For this review, take the finished solid that the model builds, in its own axes (mm). A direction names the side the tool comes from. Coordinates: 2 decimals unless noted, no trailing zeros. Write each loop counter-clockwise with the first axis right and the second up, starting at its lowest first coordinate (ties: lowest second). Pieces come first, ordered by that corner, then holes.
```python
from build123d import *

# Parameters (mm, degrees)
SKETCH_1_R      = 1
EXTRUDE_1_DEPTH = 1
FILLET_1_R      = 0.5


with BuildPart() as part:
    # 草图1 → 凸台-拉伸1 (new body)
    with BuildSketch(Plane.XY):
        with BuildLine():
            Line((-0.75, -7.095841887), (-0.75, -6.711388546))
            Line((-0.75, -6.711388546), (-0.75, -5.520914569))
            Line((-0.75, -5.520914569), (-0.75, -4.098492964))
            ThreePointArc((-0.75, -4.098492964), (-2.264950331, 2.22072913), (3.6, -0.577484586))
            ThreePointArc((3.6, -0.577484586), (2.798213716, -2.842434917), (0.75, -4.098492964))
            Line((0.75, -4.098492964), (0.75, -5.520914569))
            Line((0.75, -5.520914569), (0.75, -6.711388546))
            Line((0.75, -6.711388546), (0.75, -7.095841887))
            Line((0.75, -7.095841887), (4.616918769, -5.987758242))
            Line((4.616918769, -5.987758242), (5, -0.577484586))
            ThreePointArc((5, -0.577484586), (0, 4.422515414), (-5, -0.577484586))
            Line((-5, -0.577484586), (-4.616918769, -5.987758242))
            Line((-4.616918769, -5.987758242), (-0.75, -7.095841887))
        make_face()
        with Locations((-2.25, -4.852026876)):
            Circle(SKETCH_1_R, mode=Mode.SUBTRACT)
        with Locations((2.25, -4.852026876)):
            Circle(SKETCH_1_R, mode=Mode.SUBTRACT)
    extrude(amount=EXTRUDE_1_DEPTH)

    # 圆角1
    fillet_1_edges = [part.edges().sort_by_distance(p)[0] for p in [
        (4.616918769, -5.987758242, 0.5),
        (-4.616918769, -5.987758242, 0.5),
    ]]
    fillet(fillet_1_edges, radius=FILLET_1_R)


solid = part.part
```
Q1. Add section B-B (x = 3). State the section outline as (y, z) points, then the cut area to 3 significant figures.
Ans:
outline: (-6.45, 0) - (-5.51, 0) - (-5.51, 1) - (-6.45, 1) - close; (-4.19, 0) - (-2.57, 0) - (-2.57, 1) - (-4.19, 1) - close; (1.41, 0) - (3.42, 0) - (3.42, 1) - (1.41, 1) - close
area: 4.57 mm2
Q2. For probe 1 along Y at (x, z) = (1.75, 0.75); probe 2 along X at (y, z) = (-4.5, 0.3); probe 3 along Y at (x, z) = (-2.25, 0.55), list the stretches that pass through material, from the lowest coordinate up.
Ans:
probe 1: y = -6.81 to -5.72, -3.99 to -3.72, 2.57 to 4.11
probe 2: x = -4.72 to -3.19, -1.31 to -0.75, 0.75 to 1.31, 3.19 to 4.72
probe 3: y = -6.67 to -5.85, -3.85 to -3.39, 2.23 to 3.89
Q3. Add section D-D (z = 0.2). State the section outline as (x, y) points, then the cut area to 3 significant figures.
Ans:
outline: (-5, -0.58) - (-4.64, -5.64) arc R0.5 ccw to (-4.28, -6.08) - (-0.75, -7.1) - (-0.75, -4.1) arc R3.6 cw (long way) to (0.75, -4.1) - (0.75, -7.1) - (4.28, -6.08) arc R0.5 ccw to (4.64, -5.64) - (5, -0.58) arc R5 ccw to start; hole circle Ø2 at (-2.25, -4.85); hole circle Ø2 at (2.25, -4.85)
area: 45.8 mm2
Q4. Add section C-C (y = 0.25). State the section outline as (x, z) points, then the cut area to 3 significant figures.
Ans:
outline: (-4.93, 0) - (-3.5, 0) - (-3.5, 1) - (-4.93, 1) - close; (3.5, 0) - (4.93, 0) - (4.93, 1) - (3.5, 1) - close
area: 2.85 mm2
Q5. Add section A-A (x = 1). State the section outline as (y, z) points.
Ans:
outline: (-7.02, 0) - (-4.04, 0) - (-4.04, 1) - (-7.02, 1) - close; (2.88, 0) - (4.32, 0) - (4.32, 1) - (2.88, 1) - close
Q6. Clearance check with a flat-ended pin moving along its axis: pin 1 Ø1 at (x, y) = (-2, 0) entering from +Z. State where the tip first meets the part, or that it passes through.
Ans:
pin 1: passes through
Q7. Draft analysis for pull direction X (two halves, no side actions). For faces 3 (the cylindrical face through (-3.25, -4.81, 0.49)), 4 (the flat face through (4.82, -3.14, 0.49)), 5 (the flat face through (-2.54, -6.583, 0.493)), 6 (the flat face through (0.75, -5.6, 0.5)), state which applies: +X half, -X half, draft (parallel to the pull), parting line (faces both ways), or undercut.
Ans:
face 3: undercut
face 4: +X half
face 5: -X half
face 6: undercut
Q8. Tool access review of faces 1 (the flat face through (3, -3, 0)), 2 (the flat face through (-0.75, -5.6, 0.5)): name each direction out of +Z, -Z, +X, -X, +Y, -Y from which nothing blocks a thin tool from reaching the whole face with its end or side.
Ans:
face 1: -Z, +X, -X, +Y, -Y
face 2: +Z, -Z, -Y
